Can you work these out from the drawing? Everything is in mm from the part's minimum corner. A direction names the side the tool comes from. Coordinates: 2 decimals unless noted, no trailing zeros. Write each loop counter-clockwise with the first axis right and the second up, starting at its lowest first coordinate (ties: lowest second). Pieces come first, ordered by that corner, then holes.
(1) For pin 1 Ø1.5 at (x, y) = (12.5, 5.5) entering from +Z; pin 2 Ø2 at (y, z) = (3.5, 17) entering from +X; pin 3 Ø3 at (y, z) = (2, 23.5) entering from -X; pin 4 Ø2 at (x, y) = (11.5, 6) entering from -Z, each with a flat end and sliding along its axis, tell me the tip position at first contact or that it passes through.
(2) Please list where these lines run through material, in increasing order: probe 1 along Z at (x, y) = (1.75, 3); probe 2 along Z at (x, y) = (3.1, 3); probe 3 along Z at (x, y) = (3.75, 4.25) (1 decimal).
(3) Thinking about a two-plate mould opening in Z: for the marked faces 3, 4, 5 and 6, which applies, released by +Z, released by -Z, zero draft, split by the parting line, or undercut?
(4) Which directions (+Z, -Z, +X, -X, +Y, -Y) give clear straight access to the entire face, cutting with the end or side of a thin tool? Please do the marked faces 1 and 2.
(5) Imagine slicing it at C-C, the plane x = 3.75. List the corners of the cut face in (y, z) for me.
(6) Imagine slicing it at D-D, the plane x = 9. List the corners of the cut face in (y, z) for me, plus the area to 3 significant figures.
(7) Imagine slicing it at B-B, the plane z = 32.5. List the corners of the cut face in (x, y) for me, plus the area to 3 significant figures.
(8) Imagine slicing it at A-A, the plane x = 11.5. List the corners of the cut face in (y, z) for me, plus the area to 3 significant figures.
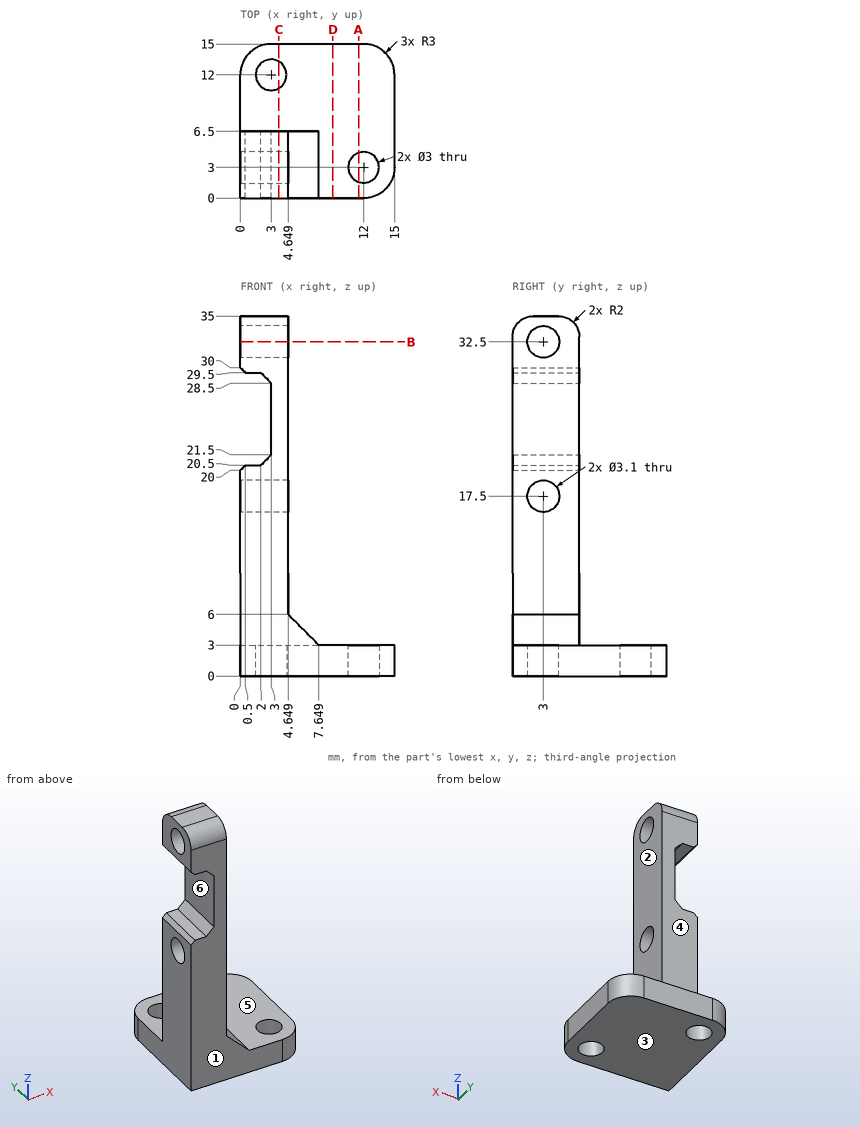
Recorded:
1. pin 1: stops at z = 3
1. pin 2: stops at x = 4.65
1. pin 3: stops at x = 3
1. pin 4: stops at z = 0
2. probe 1: z = 0 to 15.95, 19.05 to 20.5, 29.5 to 30.95, 34.05 to 35
2. probe 2: z = 0 to 15.95, 19.05 to 30.95, 34.05 to 35
2. probe 3: z = 0 to 16.6, 18.4 to 31.6, 33.4 to 35
3. face 3: released by -Z
3. face 4: zero draft
3. face 5: released by +Z
3. face 6: undercut
4. face 1: +Z, -Z, +X, -X, -Y
4. face 2: +Z, +X, +Y, -Y
5. outline: (0, 0) - (10.7, 0) - (10.7, 3) - (6.5, 3) - (6.5, 33) arc R2 ccw to (4.5, 35) - (2, 35) arc R2 ccw to (0, 33) - close; (13.3, 0) - (15, 0) - (15, 3) - (13.3, 3) - close; hole circle Ø3.1 at (3, 17.5); hole circle Ø3.1 at (3, 32.5)
6. outline: (0, 0) - (15, 0) - (15, 3) - (0, 3) - close
6. area: 45.0 mm2
7. outline: (0, 0) - (4.65, 0) - (4.65, 1.45) - (0, 1.45) - close; (0, 4.55) - (4.65, 4.55) - (4.65, 6.5) - (0, 6.5) - close
7. area: 15.8 mm2
8. outline: (0, 0) - (1.59, 0) - (1.59, 3) - (0, 3) - close; (4.41, 0) - (15, 0) - (15, 3) - (4.41, 3) - close
8. area: 36.5 mm2
